from build123d import *

# Parameters (mm, degrees)
BOSS_EXTRUDE1_DEPTH = 2
BOSS_EXTRUDE2_DEPTH = 6.5
CUT_EXTRUDE1_DEPTH  = 6.5
CUT_EXTRUDE2_DEPTH  = 6.5
BOSS_EXTRUDE3_DEPTH = 1
BOSS_EXTRUDE4_DEPTH = 1


with BuildPart() as part:
    # Sketch1 → Boss-Extrude1 (new body)
    with BuildSketch(Plane(origin=(0, 0, 0), x_dir=(0, 0, -1), z_dir=(1, 0, 0))):
        Polygon((3.15, 20), (20, 3.15), (20, 0), (0, 0), (0, 20), align=None)
    extrude(amount=BOSS_EXTRUDE1_DEPTH)

    # Sketch2 → Boss-Extrude2 (add)
    with BuildSketch(Plane(origin=(2, 0, 0), x_dir=(0, 0, -1), z_dir=(1, 0, 0))):
        Polygon((20, 0), (0, 0), (0, 3), (0, 20), (2, 20), (2, 3), (20, 3), align=None)
    extrude(amount=BOSS_EXTRUDE2_DEPTH)

    # Sketch3 → Cut-Extrude1 (cut)
    with BuildSketch(Plane.XY):
        with BuildLine():
            Line((5.5, 11.5), (5.5, 8.5))
            ThreePointArc((5.5, 8.5), (6.378679656, 6.378679656), (8.5, 5.5))
            Line((8.5, 5.5), (8.5, 14.5))
            ThreePointArc((8.5, 14.5), (6.378679656, 13.621320344), (5.5, 11.5))
        make_face()
    extrude(amount=-CUT_EXTRUDE1_DEPTH, mode=Mode.SUBTRACT)

    # Sketch4 → Cut-Extrude2 (cut)
    with BuildSketch(Plane.XZ):
        with BuildLine():
            Line((5.5, -8.5), (5.5, -11.5))
            ThreePointArc((5.5, -11.5), (6.378679656, -13.621320344), (8.5, -14.5))
            Line((8.5, -14.5), (8.5, -5.5))
            ThreePointArc((8.5, -5.5), (6.378679656, -6.378679656), (5.5, -8.5))
        make_face()
    extrude(amount=-CUT_EXTRUDE2_DEPTH, mode=Mode.SUBTRACT)

    # Sketch5 → Boss-Extrude3 (add)
    with BuildSketch(Plane(origin=(0, 0, 0), x_dir=(-1, 0, 0), z_dir=(0, -1, 0))):
        with BuildLine():
            Line((-7.5, 1.5), (-8.5, 1.5))
            Line((-8.5, 1.5), (-8.5, 3.5))
            Line((-8.5, 3.5), (-7.5, 3.5))
            ThreePointArc((-7.5, 3.5), (-6.5, 2.5), (-7.5, 1.5))
        make_face()
        with BuildLine():
            Line((-8.5, 18.5), (-8.5, 16.5))
            Line((-8.5, 16.5), (-7.5, 16.5))
            ThreePointArc((-7.5, 16.5), (-6.5, 17.5), (-7.5, 18.5))
            Line((-7.5, 18.5), (-8.5, 18.5))
        make_face()
    extrude(amount=BOSS_EXTRUDE3_DEPTH)

    # Sketch6 → Boss-Extrude4 (add)
    with BuildSketch(Plane.XY):
        with BuildLine():
            Line((7.5, 18.5), (8.5, 18.5))
            Line((8.5, 18.5), (8.5, 16.5))
            Line((8.5, 16.5), (7.5, 16.5))
            ThreePointArc((7.5, 16.5), (6.5, 17.5), (7.5, 18.5))
        make_face()
        with BuildLine():
            Line((8.5, 1.5), (8.5, 3.5))
            Line((8.5, 3.5), (7.5, 3.5))
            ThreePointArc((7.5, 3.5), (6.5, 2.5), (7.5, 1.5))
            Line((7.5, 1.5), (8.5, 1.5))
        make_face()
    extrude(amount=BOSS_EXTRUDE4_DEPTH)

    # Mirror2: part across plane


with BuildPart() as part_1:
    add(part.part)
    add(part.part.mirror(Plane(origin=(8.5, 0, 0), x_dir=(0, 0, 1), z_dir=(1, 0, 0))))


solid = part_1.part
Here's how the part is built. I have some questions about the finished solid (model axes, mm). A direction names the side the tool comes from. Coordinates: 2 decimals unless noted, no trailing zeros. Loops run counter-clockwise (first coordinate to the right, second up) from the corner with the lowest first, then second, coordinate; pieces in that order, holes last.
1. Imagine slicing it at A-A, the plane y = 2.5. Please give me the cut outline in (x, z).
2. For P1, Ø0.9, axis at y = 2, z = -10, coming from the -X side; P2, Ø2, axis at x = 14, y = 6, coming from the +Z side; P3, Ø4, axis at x = 6.5, y = 13.5, coming from the -Z side; P4, Ø4, axis at x = 9, z = -7, coming from the +Y side, each with a flat end and sliding along its axis, tell me the tip position at first contact or that it passes through.
3. If we mould it in two halves opening along X, with no side actions, what happens to faces 4 (the flat face through (5, 0, -10)), 5 (the flat face through (11.5, 1, -10)), 6 (the cylindrical face through (6.5, 17.5, 0.5))? For each: pulls with the +X half, pulls with the -X half, needs draft (parallel to the pull), parting line crosses it, or undercut.
4. I need wall thicknesses on L1, parallel to X at y = 13.75, z = -3; L2, parallel to Z at x = 13, y = 17; L3, parallel to Z at x = 16, y = 2. Which ranges of each line are inside material? Lowest first, please.
5. For faces 1 (the flat face through (8.5, 1.5, 0.5)), 2 (the flat face through (5.5, 1, -10)), 3 (the flat face through (11.5, 3, -12.9)), which set-ups out of +Z, -Z, +X, -X, +Y, -Y let a thin tool reach every point of the face, with its end or its side?
6. Imagine slicing it at C-C, the plane z = -12.25. Please give me the cut outline in (x, y).
7. Imagine slicing it at D-D, the plane y = 7. Please give me the cut outline in (x, z).
8. Imagine slicing it at B-B, the plane x = 9. Count the separate pieces of the cut face and the enclosed holes in it, and give its area (3 significant figures).
Taken from the geometry:
1. outline: (0, -20) - (17, -20) - (17, 0) - (10.5, 0) - (10.5, 1) - (6.5, 1) - (6.5, 0) - (0, 0) - close; hole (5.5, -11.5) arc R3 ccw to (11.5, -11.5) - (11.5, -8.5) arc R3 ccw to (5.5, -8.5) - close
2. P1: stops at x = 0
2. P2: stops at z = 0
2. P3: stops at z = -2
2. P4: stops at y = 3
3. face 4: needs draft
3. face 5: undercut
3. face 6: pulls with the -X half
4. L1: x = 0 to 2, 15 to 17
4. L2: z = -2 to 0
4. L3: z = -20 to 0
5. face 1: +Z, +X, -X, -Y
5. face 2: +Y, -Y
5. face 3: -Z, +Y
6. outline: (0, 0) - (5.6, 0) - (5.6, 3) - (2, 3) - (2, 10.9) - (0, 10.9) - close; (11.4, 0) - (17, 0) - (17, 10.9) - (15, 10.9) - (15, 3) - (11.4, 3) - close
7. outline: (0, -16.15) - (2, -16.15) - (2, -2) - (5.9, -2) - (5.9, 0) - (0, 0) - close; (11.1, -2) - (15, -2) - (15, -16.15) - (17, -16.15) - (17, 0) - (11.1, 0) - close
8. separate pieces: 3
8. enclosed holes: 0
8. area: 57.4 mm2
